Input: part model. Units: mm. Frame: model coordinates. Coordinates: 2 decimals unless noted, no trailing zeros. Loops run counter-clockwise (first coordinate to the right, second up) from the corner with the lowest first, then second, coordinate; pieces in that order, holes last.
```python
from build123d import *

# Parameters (mm, degrees)
SKETCH1_R           = 50.8
SKETCH1_R_2         = 19.05
BOSS_EXTRUDE1_DEPTH = 27.94
SKETCH3_R           = 9.525
BOSS_EXTRUDE3_DEPTH = 22.86
FILLET1_R           = 12.7


with BuildPart() as part:
    # Sketch1 → Boss-Extrude1 (new, symmetric)
    with BuildSketch(Plane(origin=(0, 0, 0), x_dir=(1, 0, 0), z_dir=(0, 1, 0))):
        with Locations(Location((0, 0, 0), (0, 0, 270))):
            Circle(SKETCH1_R)
        with Locations(Location((0, 0, 0), (0, 0, 270))):
            Circle(SKETCH1_R_2, mode=Mode.SUBTRACT)
    extrude(amount=BOSS_EXTRUDE1_DEPTH, both=True)

    # Sketch3 → Boss-Extrude3 (add, symmetric)
    with BuildSketch(Plane(origin=(0, 0, 0), x_dir=(1, 0, 0), z_dir=(0, 1, 0))):
        Polygon((-46.070521031, 21.404370862), (46.070521031, 21.404370862), (0, 254), align=None)
        with Locations(Location((0, 177.8, 0), (0, 0, 270))):
            Circle(SKETCH3_R, mode=Mode.SUBTRACT)
    extrude(amount=BOSS_EXTRUDE3_DEPTH, both=True)

    # Fillet1
    fillet1_edges = [part.edges().sort_by_distance(p)[0] for p in [
        (0, 0, -254),
    ]]
    fillet(fillet1_edges, radius=FILLET1_R)


solid = part.part
```
Item 1: Section query A-A (x = 0). Output: boundary loops of the cut face in (y, z) (3 decimals), then the cut area to 3 significant figures.
Result:
outline: (-27.94, -50.8) - (-22.86, -50.8) - (-22.86, -168.275) - (22.86, -168.275) - (22.86, -50.8) - (27.94, -50.8) - (27.94, -19.05) - (-27.94, -19.05) - close; (-27.94, 19.05) - (27.94, 19.05) - (27.94, 50.8) - (-27.94, 50.8) - close; (-22.86, -201.336) - (22.86, -201.336) - (22.86, -187.325) - (-22.86, -187.325) - close
area: 9,560 mm2
Item 2: Line query: L1, parallel to X at y = 20.5, z = -1; L2, parallel to Z at x = 6.5, y = 21; L3, parallel to Y at x = -19.5, z = -68. Output: solid intervals per line, ascending.
Result:
L1: x = -50.79 to -19.02, 19.02 to 50.79
L2: z = -199.55 to -184.76, -170.84 to -17.91, 17.91 to 50.38
L3: y = -22.86 to 22.86
Item 3: Section query C-C (y = -4.5). Output: boundary loops of the cut face in (x, z) (3 decimals), then the cut area to 3 significant figures.
Result:
outline: (-46.071, -21.404) - (-12.458, -191.104) arc R12.7 ccw to (12.458, -191.104) - (46.071, -21.404) arc R50.8 ccw (long way) to start; hole circle Ø38.1 at (0, 0); hole circle Ø19.05 at (0, -177.8)
area: 14,900 mm2
Item 4: Section query B-B (z = 0). Output: boundary loops of the cut face in (x, y).
Result:
outline: (-50.8, -27.94) - (-19.05, -27.94) - (-19.05, 27.94) - (-50.8, 27.94) - close; (19.05, -27.94) - (50.8, -27.94) - (50.8, 27.94) - (19.05, 27.94) - close
Item 5: Mould query, pull axis X, two halves, no side actions, for faces 1 (the face through (-29.03, 0.32, -107.44)), 2 (the face through (1, -27.94, 22)), 3 (the face through (0.419, -0.32, -187.316)). Classes: +X half, -X half, draft (parallel to the pull), parting line (faces both ways), or undercut.
Result:
face 1: -X half
face 2: draft
face 3: undercut
Item 6: Contact query for flat-ended pins moving along their axis: P1, Ø3, axis at x = 3.5, y = 9.5, coming from the +Z side; P2, Ø8, axis at y = 17, z = -173.5, coming from the -X side; P3, Ø5, axis at x = -34.5, y = 9.5, coming from the +Z side; P4, Ø11.5, axis at x = 0, z = -177.8, coming from the -Y side (3 decimals). Output: stop coordinate, or through.
Result:
P1: stops at z = 50.76
P2: stops at x = -16.74
P3: stops at z = 39.45
P4: passes through
Item 7: Section query D-D (x = 15). Output: boundary loops of the cut face in (y, z), then the cut area to 3 significant figures.
Result:
outline: (-27.94, -48.53) - (-22.86, -48.53) - (-22.86, -178.27) - (22.86, -178.27) - (22.86, -48.53) - (27.94, -48.53) - (27.94, -11.74) - (-27.94, -11.74) - close; (-27.94, 11.74) - (27.94, 11.74) - (27.94, 48.53) - (-27.94, 48.53) - close
area: 10,000 mm2
